```python
from build123d import *

# Parameters (mm, degrees)
F0_R     = 10
F0_R_2   = 1
F1_DEPTH = 1.5
F2_R     = 2.5
F2_R_2   = 1
F3_DEPTH = 3.8
F4_R     = 0.6498381819
F5_DEPTH = 1.5


# Not quite as in the source:
# - a feature names something its author has since deleted; it is built from what else it names


with BuildPart() as f1:
    # F0 (on Top) → F1 (new body)
    with BuildSketch(Plane.XY):
        Circle(F0_R)
        Circle(F0_R_2, mode=Mode.SUBTRACT)
    extrude(amount=F1_DEPTH)

    # F2 (on face) → F3 (join)
    with BuildSketch(Plane.XY.offset(1.5)):
        Circle(F2_R)
        Circle(F2_R_2, mode=Mode.SUBTRACT)
    extrude(amount=F3_DEPTH)

    # F4 (on Top) → F5 (cut, through all)
    with BuildSketch(Plane.XY):
        with Locations((0, -3.5616646055)):
            Circle(F4_R)
    extrude(amount=F5_DEPTH, mode=Mode.SUBTRACT)


solid = f1.part
```
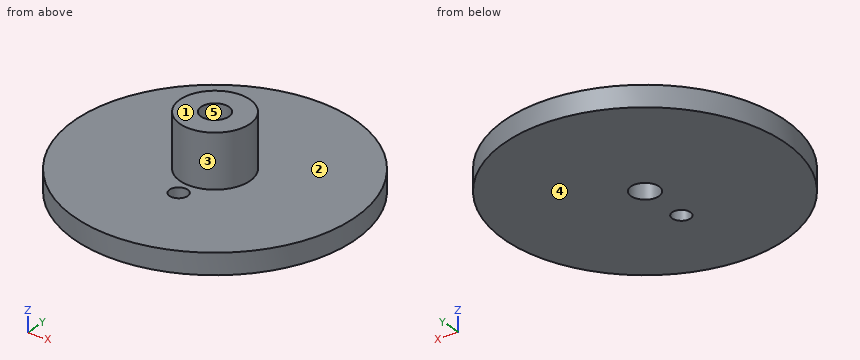
Model file for the job. Use its own axes, mm. Face numbers are marked on the shaded views. A direction names the side the tool comes from. Give positions to 0.01 mm unless a question says otherwise; leave off trailing zeros. Write each loop counter-clockwise with the first axis right and the second up, starting at its lowest first coordinate (ties: lowest second). Pieces come first, ordered by that corner, then holes. Notation, with made-up numbers: (18, 11) -> (42, 11) arc R20 cw to (42, 44) -> close; hole circle Ø7 at (-26.75, 26). An arc over 180 degrees is marked (long way). Use CSV: the item, a comma, the result in double quotes. Start each with the question number.
1) Two-plate mould, pull along X, no slides. Class the marked faces 3, 4 and 5: released by +X, released by -X, zero draft, split by the parting line, or undercut.
2) Cut at A-A on x = 0. List the corners of the cut face in (y, z).
3) Drill centre lines: L1, parallel to Y at x = 0, z = 0.65; L2, parallel to Y at x = 0, z = 2; L3, parallel to Z at x = 6.5, y = 3.75. Where is each one in solid material? Low to high.
4) Cut at C-C on z = 4.5. List the corners of the cut face in (x, y).
5) Cut at D-D on x = 3. List the corners of the cut face in (y, z), plus the area to 3 significant figures.
6) Pin check, flat tips, straight feed: P1, Ø1.5, axis at x = -1, y = 0.5, coming from the -Z side; P2, Ø1, axis at x = -2, z = 4, coming from the +Y side. Stop position of each tip, or through.
7) Tool access for the marked faces 1 and 2: list every direction of +Z, -Z, +X, -X, +Y, -Y with a clear straight run to the whole face (end or side of a thin tool).
8) Cut at B-B on y = 0. List the corners of the cut face in (x, z), plus the area to 3 significant figures.
Final values:
1,face 3,"split by the parting line"
1,face 4,"zero draft"
1,face 5,"undercut"
2,outline,"(-10, 0) -> (-4.21, 0) -> (-4.21, 1.5) -> (-10, 1.5) -> close; (-2.91, 0) -> (-1, 0) -> (-1, 5.3) -> (-2.5, 5.3) -> (-2.5, 1.5) -> (-2.91, 1.5) -> close; (1, 0) -> (10, 0) -> (10, 1.5) -> (2.5, 1.5) -> (2.5, 5.3) -> (1, 5.3) -> close"
3,L1,"y = -10 to -4.21, -2.91 to -1, 1 to 10"
3,L2,"y = -2.5 to -1, 1 to 2.5"
3,L3,"z = 0 to 1.5"
4,outline,"circle Ø5 at (0, 0); hole circle Ø2 at (0, 0)"
5,outline,"(-9.54, 0) -> (9.54, 0) -> (9.54, 1.5) -> (-9.54, 1.5) -> close"
5,area,"28.6 mm2"
6,P1,"stops at z = 0"
6,P2,"stops at y = 2"
7,face 1,"+Z, +X, -X, +Y, -Y"
7,face 2,"+Z"
8,outline,"(-10, 0) -> (-1, 0) -> (-1, 5.3) -> (-2.5, 5.3) -> (-2.5, 1.5) -> (-10, 1.5) -> close; (1, 0) -> (10, 0) -> (10, 1.5) -> (2.5, 1.5) -> (2.5, 5.3) -> (1, 5.3) -> close"
8,area,"38.4 mm2"
